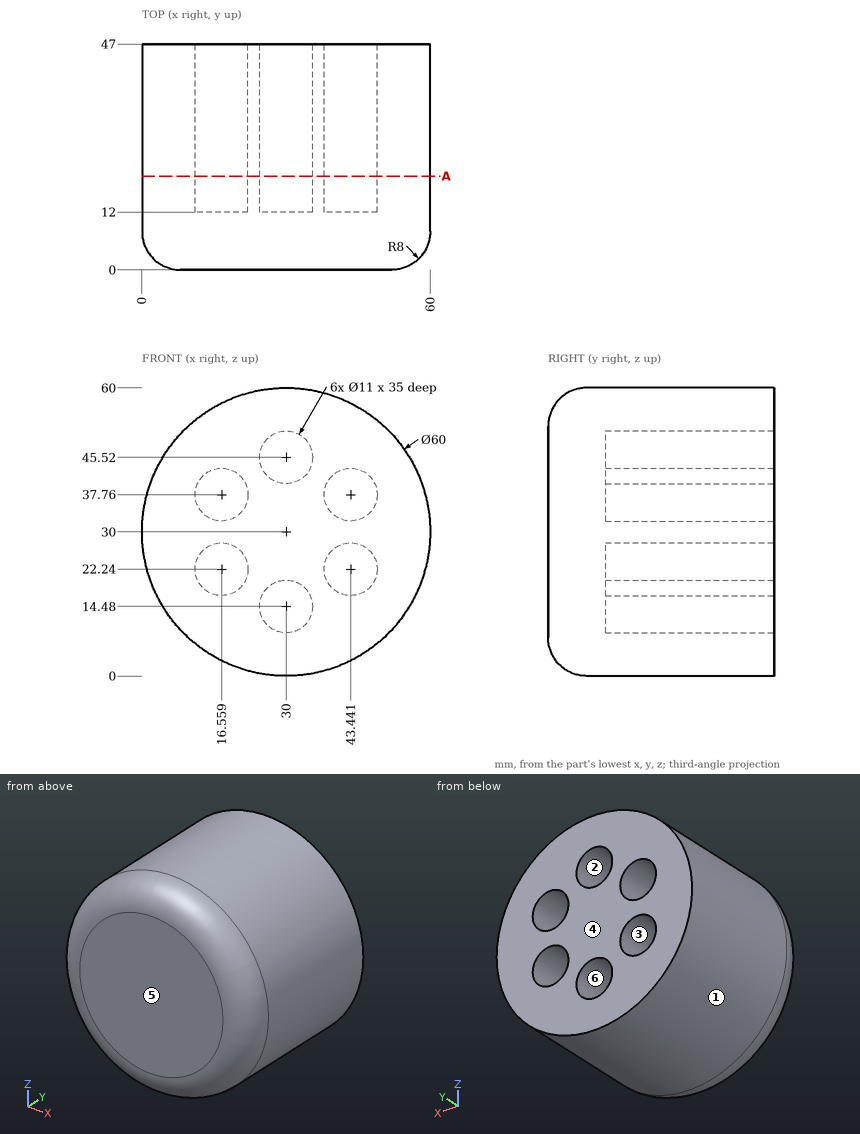
Geometry check sheet. Reference: drawing and pictorial views, mm from the part's lowest x, y, z. A direction names the side the tool comes from. Coordinates: 2 decimals unless noted, no trailing zeros. Order: outer loops, then holes, each group sorted by start corner. A loop starts at its lowest first (then second) coordinate and runs counter-clockwise, first axis right, second up. Notation, with made-up numbers: (66.5, 82) -> (79.5, 82) arc R34 ccw to (79.5, 114) -> close; hole circle Ø8 at (45, 11). An arc over 180 degrees is marked (long way). Write item = value, one per line. Start each with the question number.
1) Access from +Z, -Z, +X, -X, +Y, -Y to the whole of each face (thin tool, end or side, straight path). Record for the marked faces 5 and 6.
2) Cross-section at A-A (y = 19.5). Enter the section's corners in (x, z).
3) Material ranges on L1, parallel to Z at x = 30, y = 30; L2, parallel to Z at x = 13, y = 33; L3, parallel to X at y = 25.5, z = 25, recorded low to high.
4) Go/stop test with flat-tipped pins: P1, Ø12, axis at x = 15.5, z = 36, coming from the +Y side; P2, Ø3.5, axis at x = 30.5, z = 44, coming from the +Y side; P3, Ø10, axis at x = 11.5, y = 38, coming from the -Z side; P4, Ø5, axis at y = 22.5, z = 42, coming from the +X side. Record where each tip stops, or that it passes through.
5) Mould release check, pull along Z, two halves, no side actions. Record for the marked faces 1, 2, 3 and 4: +Z half, -Z half, draft (parallel to the pull), parting line (faces both ways), or undercut.
Ans:
q1.face_5 = +Z, -Z, +X, -X, -Y
q1.face_6 = +Y
q2.outline = circle Ø60 at (30, 30); hole circle Ø11 at (16.56, 22.24); hole circle Ø11 at (16.56, 37.76); hole circle Ø11 at (30, 14.48); hole circle Ø11 at (30, 45.52); hole circle Ø11 at (43.44, 22.24); hole circle Ø11 at (43.44, 37.76)
q3.L1 = 0 to 8.98, 19.98 to 40.02, 51.02 to 60
q3.L2 = 5.28 to 18.05, 26.43 to 33.57, 41.95 to 54.72
q3.L3 = 0.42 to 11.8, 21.32 to 38.68, 48.2 to 59.58
q4.P1 = 47
q4.P2 = 12
q4.P3 = 3.21
q4.P4 = 58.46
q5.face_1 = parting line
q5.face_2 = undercut
q5.face_3 = undercut
q5.face_4 = draft
